Could you check a few things on this model? Use its own coordinates, in mm. A direction names the side the tool comes from. Round coordinates to 2 decimals unless told otherwise and drop trailing zeros. Write each loop counter-clockwise with the first axis right and the second up, starting at its lowest first coordinate (ties: lowest second). Pieces come first, ordered by that corner, then holes. Notation, with made-up numbers: (-15.75, 19.5) - (42.25, 19.5) arc R14 cw to (42.25, 27.5) - close; hole circle Ø10 at (25.5, -30.5). An arc over 180 degrees is marked (long way). Put each result on its own line as item: value.
from build123d import *

# Parameters (mm, degrees)
F0_W         = 40
F0_H         = 70
F1_DEPTH     = 7
F2_R         = 5
F3_R         = 1.780942195
F4_DEPTH     = 3.7
F5_T1_DEPTH  = 60
F5_T3_DEPTH  = 30
F5_T6_ANGLE  = 90
F5_T8_ANGLE  = 90
F5_T10_ANGLE = 90
F5_T12_ANGLE = 90
F5_T14_ANGLE = 90
F5_T16_ANGLE = 90
F5_T18_ANGLE = 90
F5_T20_ANGLE = 90
F6_R         = 3
F7_DEPTH     = 1
F8_W         = 24.7989948839
F8_H         = 41.9472400099
F9_DEPTH     = 4
F10_R        = 3.0419567341
F11_DEPTH    = 1.9


# Not quite as in the source:
# - a fillet or chamfer that OpenCascade refuses, or shapes differently, is made with other operations: its cross-section is extruded or revolved along the edge and cut away or added


with BuildPart() as f1:
    # F0 (on Top) → F1 (new body)
    with BuildSketch(Plane.XY):
        with Locations((20, 35)):
            Rectangle(F0_W, F0_H)
    extrude(amount=F1_DEPTH)

    # F2
    f2_edges = [f1.edges().sort_by_distance(p)[0] for p in [
        (0, 0, 3.5),
        (40, 0, 3.5),
        (40, 70, 3.5),
        (0, 70, 3.5),
    ]]
    fillet(f2_edges, radius=F2_R)

    # F3 (on face) → F4 (cut)
    with BuildSketch(Plane(origin=(0, 70, 0), x_dir=(-1, 0, 0), z_dir=(0, 1, 0))):
        with Locations((-29.880721122, 3.5)):
            Circle(F3_R)
    extrude(amount=-F4_DEPTH, mode=Mode.SUBTRACT)

    # F5: fillet of radius 2 on 16 edges, made by hand

    # F5_s2 → F5_t1 (cut)
    with BuildSketch(Plane.XZ.offset(-65)):
        with BuildLine():
            ThreePointArc((38, 0), (39.4142135624, 0.5857864376), (40, 2))
            Line((40, 2), (40, 0))
            Line((40, 0), (38, 0))
        make_face()
        with BuildLine():
            ThreePointArc((38, 7), (39.4142135624, 6.4142135624), (40, 5))
            Line((40, 5), (40, 7))
            Line((40, 7), (38, 7))
        make_face()
        with BuildLine():
            ThreePointArc((0, 2), (0.5857864376, 0.5857864376), (2, 0))
            Line((2, 0), (0, 0))
            Line((0, 0), (0, 2))
        make_face()
        with BuildLine():
            ThreePointArc((0, 5), (0.5857864376, 6.4142135624), (2, 7))
            Line((2, 7), (0, 7))
            Line((0, 7), (0, 5))
        make_face()
    extrude(amount=F5_T1_DEPTH, mode=Mode.SUBTRACT)

    # F5_s4 → F5_t3 (cut)
    with BuildSketch(Plane.YZ.offset(5)):
        with BuildLine():
            ThreePointArc((68, 0), (69.4142135624, 0.5857864376), (70, 2))
            Line((70, 2), (70, 0))
            Line((70, 0), (68, 0))
        make_face()
        with BuildLine():
            ThreePointArc((2, 0), (0.5857864376, 0.5857864376), (0, 2))
            Line((0, 2), (0, 0))
            Line((0, 0), (2, 0))
        make_face()
        with BuildLine():
            ThreePointArc((68, 7), (69.4142135624, 6.4142135624), (70, 5))
            Line((70, 5), (70, 7))
            Line((70, 7), (68, 7))
        make_face()
        with BuildLine():
            ThreePointArc((2, 7), (0.5857864376, 6.4142135624), (0, 5))
            Line((0, 5), (0, 7))
            Line((0, 7), (2, 7))
        make_face()
    extrude(amount=F5_T3_DEPTH, mode=Mode.SUBTRACT)

    # F5_s5 → F5_t6 (revolve, cut)
    with BuildSketch(Plane.XZ.offset(-65)):
        with BuildLine():
            ThreePointArc((2, 0), (0.5857864376, 0.5857864376), (0, 2))
            Line((0, 2), (0, 0))
            Line((0, 0), (2, 0))
        make_face()
    revolve(axis=Axis((5, 65, 0), (0, 0, -1)), revolution_arc=F5_T6_ANGLE, mode=Mode.SUBTRACT)

    # F5_s7 → F5_t8 (revolve, cut)
    with BuildSketch(Plane.XZ.offset(-5)):
        with BuildLine():
            ThreePointArc((2, 0), (0.5857864376, 0.5857864376), (0, 2))
            Line((0, 2), (0, 0))
            Line((0, 0), (2, 0))
        make_face()
    revolve(axis=Axis((5, 5, 0), (0, 0, 1)), revolution_arc=F5_T8_ANGLE, mode=Mode.SUBTRACT)

    # F5_s9 → F5_t10 (revolve, cut)
    with BuildSketch(Plane.XZ.offset(-65)):
        with BuildLine():
            ThreePointArc((38, 0), (39.4142135624, 0.5857864376), (40, 2))
            Line((40, 2), (40, 0))
            Line((40, 0), (38, 0))
        make_face()
    revolve(axis=Axis((35, 65, 0), (0, 0, 1)), revolution_arc=F5_T10_ANGLE, mode=Mode.SUBTRACT)

    # F5_s11 → F5_t12 (revolve, cut)
    with BuildSketch(Plane.YZ.offset(35)):
        with BuildLine():
            ThreePointArc((2, 0), (0.5857864376, 0.5857864376), (0, 2))
            Line((0, 2), (0, 0))
            Line((0, 0), (2, 0))
        make_face()
    revolve(axis=Axis((35, 5, 0), (0, 0, 1)), revolution_arc=F5_T12_ANGLE, mode=Mode.SUBTRACT)

    # F5_s13 → F5_t14 (revolve, cut)
    with BuildSketch(Plane.XZ.offset(-65)):
        with BuildLine():
            ThreePointArc((0, 5), (0.5857864376, 6.4142135624), (2, 7))
            Line((2, 7), (0, 7))
            Line((0, 7), (0, 5))
        make_face()
    revolve(axis=Axis((5, 65, 7), (0, 0, -1)), revolution_arc=F5_T14_ANGLE, mode=Mode.SUBTRACT)

    # F5_s15 → F5_t16 (revolve, cut)
    with BuildSketch(Plane.XZ.offset(-5)):
        with BuildLine():
            ThreePointArc((0, 5), (0.5857864376, 6.4142135624), (2, 7))
            Line((2, 7), (0, 7))
            Line((0, 7), (0, 5))
        make_face()
    revolve(axis=Axis((5, 5, 7), (0, 0, 1)), revolution_arc=F5_T16_ANGLE, mode=Mode.SUBTRACT)

    # F5_s17 → F5_t18 (revolve, cut)
    with BuildSketch(Plane.XZ.offset(-65)):
        with BuildLine():
            ThreePointArc((38, 7), (39.4142135624, 6.4142135624), (40, 5))
            Line((40, 5), (40, 7))
            Line((40, 7), (38, 7))
        make_face()
    revolve(axis=Axis((35, 65, 7), (0, 0, 1)), revolution_arc=F5_T18_ANGLE, mode=Mode.SUBTRACT)

    # F5_s19 → F5_t20 (revolve, cut)
    with BuildSketch(Plane.YZ.offset(35)):
        with BuildLine():
            ThreePointArc((2, 7), (0.5857864376, 6.4142135624), (0, 5))
            Line((0, 5), (0, 7))
            Line((0, 7), (2, 7))
        make_face()
    revolve(axis=Axis((35, 5, 7), (0, 0, 1)), revolution_arc=F5_T20_ANGLE, mode=Mode.SUBTRACT)

    # F6 (on face) → F7 (cut)
    with BuildSketch(Plane.XY.offset(7)):
        with Locations((20, 8.8619329035)):
            Circle(F6_R)
    extrude(amount=-F7_DEPTH, mode=Mode.SUBTRACT)

    # F8 (on face) → F9 (cut)
    with BuildSketch(Plane.XY.offset(7)):
        with Locations((21.6991202906, 38.8473635539)):
            Rectangle(F8_W, F8_H)
    extrude(amount=-F9_DEPTH, mode=Mode.SUBTRACT)

    # F10 (on face) → F11 (join)
    with BuildSketch(Plane.XY.offset(7)):
        with Locations((5.6223799475, 12.1855456382)):
            Circle(F10_R)
    extrude(amount=F11_DEPTH)


solid = f1.part
(1) Imagine slicing it at B-B, the plane x = 20. List the corners of the cut face in (y, z) for me.
Values found:
outline: (0, 2) arc R2 ccw to (2, 0) - (68, 0) arc R2 ccw to (70, 2) - (70, 5) arc R2 ccw to (68, 7) - (59.82, 7) - (59.82, 3) - (17.87, 3) - (17.87, 7) - (11.86, 7) - (11.86, 6) - (5.86, 6) - (5.86, 7) - (2, 7) arc R2 ccw to (0, 5) - close
(2) I'm going to push flat-ended pins straight in: pin 1 (1 mm diameter, centred on x = 8.5, y = 17, fed in from +Z); pin 2 (6 mm diameter, centred on x = 16, y = 38.5, fed in from +Z). Where does each tip first touch, or does it pass through?
Values found:
pin 1: stops at z = 7
pin 2: stops at z = 3
(3) For faces 1 (the face through (7.26, 14.75, 7.94)), 2 (the face through (30, 66.3, 4)), 3 (the face through (39, 68, 4)), which set-ups out of +Z, -Z, +X, -X, +Y, -Y let a thin tool reach every point of the face, with its end or its side?
Values found:
face 1: +Z
face 2: +Y
face 3: +Z, -Z, +X, +Y
(4) Imagine slicing it at A-A, the plane y = 40. List the corners of the cut face in (x, z) for me, then the cut area to 3 significant figures.
Values found:
outline: (0, 2) arc R2 ccw to (2, 0) - (38, 0) arc R2 ccw to (40, 2) - (40, 5) arc R2 ccw to (38, 7) - (34.1, 7) - (34.1, 3) - (9.3, 3) - (9.3, 7) - (2, 7) arc R2 ccw to (0, 5) - close
area: 177 mm^2
(5) Please list where these lines run through material, in increasing order: probe 1 along X at (y, z) = (69, 3.5); probe 2 along Y at (x, z) = (20, 6.35); probe 3 along Z at (x, y) = (22.5, 57). Write a range as from..to.
Values found:
probe 1: x = 2..28.1, 31.66..38
probe 2: y = 0.52..5.86, 11.86..17.87, 59.82..69.48
probe 3: z = 0..3
(6) Imagine slicing it at D-D, the plane x = 6.5. List the corners of the cut face in (y, z) for me, then the cut area to 3 significant figures.
Values found:
outline: (0, 2) arc R2 ccw to (2, 0) - (68, 0) arc R2 ccw to (70, 2) - (70, 5) arc R2 ccw to (68, 7) - (15.1, 7) - (15.1, 8.9) - (9.27, 8.9) - (9.27, 7) - (2, 7) arc R2 ccw to (0, 5) - close
area: 498 mm^2
(7) Imagine slicing it at C-C, the plane z = 8. List the corners of the cut face in (x, y) for me, then the cut area to 3 significant figures.
Values found:
outline: circle Ø6.08 at (5.62, 12.19)
area: 29.1 mm^2
(8) If we mould it in two halves opening along X, with no side actions, what happens to faces 4 (the face through (1, 68, 4)), 5 (the face through (17.8, 10.9, 6.5)), 6 (the face through (40, 35, 3)), 7 (the face through (9.3, 39, 5))? For each: pulls with the +X half, pulls with the -X half, needs draft (parallel to the pull), parting line crosses it, or undercut.
Values found:
face 4: pulls with the -X half
face 5: undercut
face 6: pulls with the +X half
face 7: undercut
